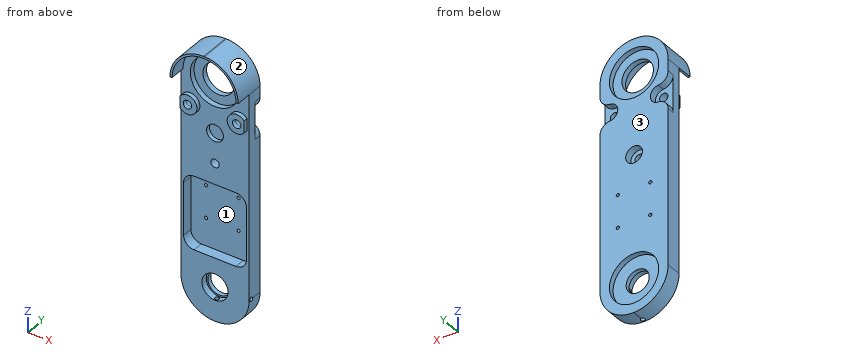
from build123d import *

# Parameters (mm, degrees)
BOSS_EXTRUDE1_DEPTH = 15
SKETCH2_R           = 23.5
CUT_EXTRUDE1_DEPTH  = 5
SKETCH3_R           = 11
CUT_EXTRUDE2_DEPTH  = 135.373546504
SKETCH17_R          = 23.5
CUT_EXTRUDE10_DEPTH = 5
SKETCH18_R          = 15
CUT_EXTRUDE11_DEPTH = 135.373546504
CUT_EXTRUDE12_START = -5
SKETCH19_R          = 23.5
CUT_EXTRUDE12_DEPTH = 5
CUT_EXTRUDE13_DEPTH = 10
SKETCH21_R          = 1.5
CUT_EXTRUDE14_DEPTH = 135.373546504
SKETCH22_R          = 8
CUT_EXTRUDE15_DEPTH = 4
SKETCH23_R          = 4
BOSS_EXTRUDE6_DEPTH = 4
SKETCH24_R          = 4
CUT_EXTRUDE16_DEPTH = 135.837865602
BOSS_EXTRUDE8_START = 15
BOSS_EXTRUDE8_DEPTH = 15
SKETCH28_R          = 8
CUT_EXTRUDE17_DEPTH = 7
FILLET1_R           = 10
SKETCH29_R          = 12.5
CUT_EXTRUDE18_DEPTH = 6
SKETCH30_R          = 2
CUT_EXTRUDE19_DEPTH = 25
SKETCH32_R          = 2
CUT_EXTRUDE20_DEPTH = 25


with BuildPart() as part:
    # Sketch1 → Boss-Extrude1 (new body)
    with BuildSketch(Plane(origin=(0, 0, 0), x_dir=(1, 0, 0), z_dir=(0, 1, 0))):
        with BuildLine():
            Line((0, 130), (0.5, 130))
            ThreePointArc((0.5, 130), (23.127416998, 120.627416998), (32.5, 98))
            Line((32.5, 98), (32.5, -98))
            ThreePointArc((32.5, -98), (23.127416998, -120.627416998), (0.5, -130))
            Line((0.5, -130), (-0.5, -130))
            ThreePointArc((-0.5, -130), (-23.127416998, -120.627416998), (-32.5, -98))
            Line((-32.5, -98), (-32.5, 97.5))
            ThreePointArc((-32.5, 97.5), (-22.980970389, 120.480970389), (0, 130))
        make_face()
    extrude(amount=BOSS_EXTRUDE1_DEPTH)

    # Sketch2 → Cut-Extrude1 (cut)
    with BuildSketch(Plane(origin=(0, 15, 0), x_dir=(1, 0, 0), z_dir=(0, 1, 0))):
        with Locations(Location((0, 97.5, 0), (0, 0, 270))):
            Circle(SKETCH2_R)
    extrude(amount=-CUT_EXTRUDE1_DEPTH, mode=Mode.SUBTRACT)

    # Sketch3 → Cut-Extrude2 (cut, through all)
    with BuildSketch(Plane(origin=(0, 10, 0), x_dir=(1, 0, 0), z_dir=(0, 1, 0))):
        with Locations(Location((0, 97.5, 0), (0, 0, 270))):
            Circle(SKETCH3_R)
    extrude(amount=-CUT_EXTRUDE2_DEPTH, mode=Mode.SUBTRACT)

    # Sketch17 → Cut-Extrude10 (cut)
    with BuildSketch(Plane.XZ):
        with Locations(Location((0, 97.5, 0), (0, 0, 270))):
            Circle(SKETCH17_R)
    extrude(amount=-CUT_EXTRUDE10_DEPTH, mode=Mode.SUBTRACT)

    # Sketch18 → Cut-Extrude11 (cut, through all)
    with BuildSketch(Plane.XZ.offset(-5)):
        with Locations(Location((0, 97.5, 0), (0, 0, 270))):
            Circle(SKETCH18_R)
    extrude(amount=-CUT_EXTRUDE11_DEPTH, mode=Mode.SUBTRACT)

    # Sketch19 → Cut-Extrude12 (cut)
    with BuildSketch(Plane(origin=(0, 15, 0), x_dir=(1, 0, 0), z_dir=(0, 1, 0)).offset(CUT_EXTRUDE12_START)):
        with Locations(Location((0, -97.5, 0), (0, 0, 90))):
            Circle(SKETCH19_R)
    extrude(amount=CUT_EXTRUDE12_DEPTH, mode=Mode.SUBTRACT)

    # Sketch20 → Cut-Extrude13 (cut)
    with BuildSketch(Plane.XZ):
        with BuildLine():
            Line((-20, 0), (20, 0))
            ThreePointArc((20, 0), (27.071067812, -2.928932188), (30, -10))
            Line((30, -10), (30, -60))
            ThreePointArc((30, -60), (27.071067812, -67.071067812), (20, -70))
            Line((20, -70), (-20, -70))
            ThreePointArc((-20, -70), (-27.071067812, -67.071067812), (-30, -60))
            Line((-30, -60), (-30, -10))
            ThreePointArc((-30, -10), (-27.071067812, -2.928932188), (-20, 0))
        make_face()
    extrude(amount=-CUT_EXTRUDE13_DEPTH, mode=Mode.SUBTRACT)

    # Sketch21 → Cut-Extrude14 (cut, through all)
    with BuildSketch(Plane.XZ.offset(-10)):
        with Locations(Location((-15.5, -12.5, 0), (0, 0, 270))):
            Circle(SKETCH21_R)
        with Locations(Location((15.5, -12.5, 0), (0, 0, 270))):
            Circle(SKETCH21_R)
        with Locations(Location((-15.5, -43.5, 0), (0, 0, 270))):
            Circle(SKETCH21_R)
        with Locations(Location((15.5, -43.5, 0), (0, 0, 270))):
            Circle(SKETCH21_R)
    extrude(amount=-CUT_EXTRUDE14_DEPTH, mode=Mode.SUBTRACT)

    # Sketch22 → Cut-Extrude15 (cut)
    with BuildSketch(Plane.XZ):
        with Locations(Location((0, 48.75, 0), (0, 0, 270))):
            Circle(SKETCH22_R)
    extrude(amount=-CUT_EXTRUDE15_DEPTH, mode=Mode.SUBTRACT)

    # Sketch23 → Boss-Extrude6 (add)
    # profile 1 of 2: a face of its own
    with BuildSketch(Plane.XZ):
        with BuildLine():
            Line((-30.5, 74.616516124), (-30.5, 62.993052049))
            ThreePointArc((-30.5, 62.993052049), (-14.401855723, 68.804784086), (-30.5, 74.616516124))
        make_face()
        with Locations(Location((-23.5, 68.804784086, 0), (0, 0, 270))):
            Circle(SKETCH23_R, mode=Mode.SUBTRACT)
    # profile 2 of 2: a face of its own
    with BuildSketch(Plane.XZ):
        with BuildLine():
            Line((30.5, 74.616516124), (30.5, 62.993052049))
            ThreePointArc((30.5, 62.993052049), (14.401855723, 68.804784086), (30.5, 74.616516124))
        make_face()
        with Locations(Location((23.5, 68.804784086, 0), (0, 0, 90))):
            Circle(SKETCH23_R, mode=Mode.SUBTRACT)
    extrude(amount=BOSS_EXTRUDE6_DEPTH)

    # Sketch24 → Cut-Extrude16 (cut, through all)
    with BuildSketch(Plane.XZ):
        with Locations(Location((0, 20, 0), (0, 0, 270))):
            Circle(SKETCH24_R)
        with Locations(Location((-23.5, 68.804784086, 0), (0, 0, 270))):
            Circle(SKETCH24_R)
        with Locations(Location((23.5, 68.804784086, 0), (0, 0, 90))):
            Circle(SKETCH24_R)
    extrude(amount=-CUT_EXTRUDE16_DEPTH, mode=Mode.SUBTRACT)

    # Sketch27 → Boss-Extrude8 (add)
    with BuildSketch(Plane.XZ.offset(BOSS_EXTRUDE8_START)):
        with BuildLine():
            Line((-0.5, 128), (0.5, 128))
            ThreePointArc((0.5, 128), (21.713203436, 119.213203436), (30.5, 98))
            Line((30.5, 98), (32.5, 98))
            ThreePointArc((32.5, 98), (23.127416998, 120.627416998), (0.5, 130))
            Line((0.5, 130), (-0.5, 130))
            ThreePointArc((-0.5, 130), (-23.127416998, 120.627416998), (-32.5, 98))
            Line((-32.5, 98), (-30.5, 98))
            ThreePointArc((-30.5, 98), (-21.713203436, 119.213203436), (-0.5, 128))
        make_face()
    extrude(amount=-BOSS_EXTRUDE8_DEPTH)

    # Sketch28 → Cut-Extrude17 (cut)
    with BuildSketch(Plane(origin=(0, 15, 0), x_dir=(1, 0, 0), z_dir=(0, 1, 0))):
        with Locations(Location((0, -20, 0), (0, 0, 270))):
            Circle(SKETCH28_R)
        with BuildLine():
            Line((-23.5, -60.804784086), (-32.5, -60.804784086))
            Line((-32.5, -60.804784086), (-32.5, -76.804784086))
            Line((-32.5, -76.804784086), (-23.5, -76.804784086))
            ThreePointArc((-23.5, -76.804784086), (-15.5, -68.804784086), (-23.5, -60.804784086))
        make_face()
        with BuildLine():
            Line((32.5, -60.804784086), (32.5, -76.804784086))
            Line((32.5, -76.804784086), (23.5, -76.804784086))
            ThreePointArc((23.5, -76.804784086), (15.5, -68.804784086), (23.5, -60.804784086))
            Line((23.5, -60.804784086), (32.5, -60.804784086))
        make_face()
    extrude(amount=-CUT_EXTRUDE17_DEPTH, mode=Mode.SUBTRACT)

    # Fillet1
    # the kernel refuses this fillet: 10 mm, written as the material it takes off along each edge
    with BuildSketch(Plane(origin=(32.5, 39.930501889, 76.804784086), x_dir=(0, 0, 1), z_dir=(0, -1, 0)), Plane(origin=(-32.5, 39.930501889, 60.804784086), x_dir=(0, 0, -1), z_dir=(0, -1, 0))) as fillet1_piece_1:
        with BuildLine():
            CenterArc((9.972200756, 10), FILLET1_R, 183.184738537, 86.815261463)
            Line((-0.01235522, 9.444444444), (-1.010810817, 9.388888889))
            ThreePointArc((-1.010810817, 9.388888889), (-1, 9), (-1, 0))
            Line((-1, 0), (0, -1))
            Line((0, -1), (9.972200756, -1))
            Line((9.972200756, -1), (9.972200756, 0))
        make_face()
    extrude(amount=31.930501889, mode=Mode.SUBTRACT)
    with BuildSketch(Plane(origin=(32.5, 39.930501889, 60.804784086), x_dir=(0, 0, -1), z_dir=(0, -1, 0)), Plane(origin=(-32.5, 39.930501889, 76.804784086), x_dir=(0, 0, 1), z_dir=(0, -1, 0))) as fillet1_piece_2:
        with BuildLine():
            CenterArc((9.972200756, -10), FILLET1_R, 90, 86.815261463)
            Line((-0.01235522, -9.444444444), (-1.010810817, -9.388888889))
            ThreePointArc((-1.010810817, -9.388888889), (-1, -9), (-1, 0))
            Line((-1, 0), (0, 1))
            Line((0, 1), (9.972200756, 1))
            Line((9.972200756, 1), (9.972200756, 0))
        make_face()
    extrude(amount=31.930501889, mode=Mode.SUBTRACT)

    # Sketch29 → Cut-Extrude18 (cut)
    with BuildSketch(Plane.XZ):
        with Locations(Location((0, -97.5, 0), (0, 0, 270))):
            Circle(SKETCH29_R)
    extrude(amount=-CUT_EXTRUDE18_DEPTH, mode=Mode.SUBTRACT)

    # Sketch30 → Cut-Extrude19 (cut)
    with BuildSketch(Plane(origin=(0, 0, -130), x_dir=(-1, 0, 0), z_dir=(0, 0, -1))):
        with Locations(Location((0, 3, 0), (0, 0, 270))):
            Circle(SKETCH30_R)
    extrude(amount=-CUT_EXTRUDE19_DEPTH, mode=Mode.SUBTRACT)

    # Sketch32 → Cut-Extrude20 (cut)
    with BuildSketch(Plane(origin=(32.5, 0, 0), x_dir=(0, 0, -1), z_dir=(1, 0, 0))):
        with Locations((98, 3)):
            Circle(SKETCH32_R)
    extrude(amount=-CUT_EXTRUDE20_DEPTH, mode=Mode.SUBTRACT)


solid = part.part
Geometry: final body of the model. Coordinates: model frame, mm. Face numbers are marked on the shaded views. Give positions to 0.01 mm unless a question says otherwise; leave off trailing zeros. Write each loop counter-clockwise with the first axis right and the second up, starting at its lowest first coordinate (ties: lowest second). Pieces come first, ordered by that corner, then holes. Notation, with made-up numbers: (-34, 16) -> (-30, 16) arc R15 ccw to (-30, 42) -> close; hole circle Ø7 at (40.5, 5). An arc over 180 degrees is marked (long way). Answer as a JSON object with one key per item and string values.
1. Ray query, probe 1 along X at (y, z) = (12.3, -12.5); probe 2 along Z at (x, y) = (13, 11); probe 3 along Z at (x, y) = (-13, 5.5). Return the intervals inside material, ascending. Write a range as from..to.
Ans:
{"probe 1": "x = -32.5..-17, -14..14, 17..32.5", "probe 2": "z = -127.46..-117.08, -77.92..77.92, 117.08..127.46", "probe 3": "z = -127.29..-70, 0..90.02, 104.98..127.46"}
2. Mould query, pull axis Z, two halves, no side actions, for the marked faces 1, 2 and 3. Classes: pulls with the +Z half, pulls with the -Z half, needs draft (parallel to the pull), parting line crosses it, or undercut.
Ans:
{"face 1": "undercut", "face 2": "pulls with the +Z half", "face 3": "needs draft"}
3. Contact query for flat-ended pins moving along their axis: pin 1 (17.5 mm diameter, centred on x = -24, z = 69, fed in from -Y); pin 2 (14.5 mm diameter, centred on x = 0, z = 20, fed in from +Y); pin 3 (1.5 mm diameter, centred on x = -23.5, y = -10, fed in from +Z). Output: stop coordinate, or through.
Ans:
{"pin 1": "stops at y = -4", "pin 2": "stops at y = 8", "pin 3": "stops at z = 121"}
4. Cut plane D-D on z = -17. Output: boundary loops of the cut face in (x, y), and give its area (3 significant figures).
Ans:
{"outline": "(-32.5, 0) -> (-30, 0) -> (-30, 10) -> (30, 10) -> (30, 0) -> (32.5, 0) -> (32.5, 15) -> (-32.5, 15) -> close", "area": "375 mm^2"}
5. Cut plane A-A on z = 20. Output: boundary loops of the cut face in (x, y), and give its area (3 significant figures).
Ans:
{"outline": "(-32.5, 0) -> (-4, 0) -> (-4, 8) -> (-8, 8) -> (-8, 15) -> (-32.5, 15) -> close; (4, 0) -> (32.5, 0) -> (32.5, 15) -> (8, 15) -> (8, 8) -> (4, 8) -> close", "area": "799 mm^2"}
6. Cut plane B-B on y = 12.5. Output: boundary loops of the cut face in (x, z), and give its area (3 significant figures).
Ans:
{"outline": "(-32.5, -97.5) arc R32.5 ccw to (0, -130) -> (0.5, -130) arc R32 ccw to (32.5, -98) -> (32.5, 50.83) arc R10 ccw to (23.06, 60.82) arc R8 cw to (23.06, 76.79) arc R10 ccw to (32.5, 86.78) -> (32.5, 98) arc R32 ccw to (0.5, 130) -> (-0.5, 130) arc R32 ccw to (-32.5, 98) -> (-32.5, 86.78) arc R10 ccw to (-23.06, 76.79) arc R8 cw to (-23.06, 60.82) arc R10 ccw to (-32.5, 50.83) -> close; hole circle Ø47 at (0, -97.5); hole circle Ø47 at (0, 97.5); hole circle Ø3 at (-15.5, -43.5); hole circle Ø3 at (-15.5, -12.5); hole circle Ø16 at (0, 20); hole circle Ø3 at (15.5, -43.5); hole circle Ø3 at (15.5, -12.5)", "area": "11,700 mm^2"}
7. Cut plane C-C on y = -9. Output: boundary loops of the cut face in (x, z).
Ans:
{"outline": "(-32.5, 98) -> (-30.5, 98) arc R30 cw to (-0.5, 128) -> (0.5, 128) arc R30 cw to (30.5, 98) -> (32.5, 98) arc R32 ccw to (0.5, 130) -> (-0.5, 130) arc R32 ccw to start"}
